The model under review builds one solid part; all positions refer to its coordinate system, in mm. Face numbers are marked on the shaded views. A direction names the side the tool comes from. Give positions to 0.01 mm unless a question says otherwise; leave off trailing zeros. Loops run counter-clockwise (first coordinate to the right, second up) from the corner with the lowest first, then second, coordinate; pieces in that order, holes last. Notation, with made-up numbers: (30.25, -26) - (51.25, -26) arc R20 cw to (51.25, -3) - close; hole circle Ø7 at (55.5, 19). An arc over 180 degrees is marked (long way). Answer as a JSON object with one key per item and string values.
from build123d import *

# Parameters (mm, degrees)
BOSS_EXTRUDE1_DEPTH = 100
SKETCH3_W           = 6
SKETCH3_H           = 6
BOSS_EXTRUDE2_DEPTH = 6
SKETCH4_R           = 1
CUT_EXTRUDE2_DEPTH  = 10
SKETCH5_R           = 1
CUT_EXTRUDE3_DEPTH  = 10
FILLET1_R           = 1
FILLET2_R           = 2
SKETCH7_W           = 11
SKETCH7_H           = 5.6
CUT_EXTRUDE4_DEPTH  = 10
SKETCH13_W          = 6
SKETCH13_H          = 6
BOSS_EXTRUDE3_DEPTH = 6
SKETCH14_R          = 1
CUT_EXTRUDE7_DEPTH  = 6
SKETCH16_R          = 1
CUT_EXTRUDE8_DEPTH  = 6
FILLET3_R           = 2
FILLET4_R           = 1
BOSS_EXTRUDE4_DEPTH = 5
BOSS_EXTRUDE5_DEPTH = 5
SKETCH19_W          = 0.937777778
SKETCH19_H          = 14.2
BOSS_EXTRUDE6_DEPTH = 10
SKETCH20_W          = 0.937777778
SKETCH20_H          = 14.2
BOSS_EXTRUDE7_DEPTH = 10
SKETCH21_W          = 2
SKETCH21_H          = 2.5
BOSS_EXTRUDE8_DEPTH = 1
SKETCH22_W          = 2
SKETCH22_H          = 2.5
BOSS_EXTRUDE9_DEPTH = 1


with BuildPart() as part:
    # Sketch1 → Boss-Extrude1 (new body)
    with BuildSketch(Plane.XY):
        Polygon((0, 0), (10, 0), (2, 45), (0, 45), align=None)
    extrude(amount=BOSS_EXTRUDE1_DEPTH)

    # Sketch3 → Boss-Extrude2 (add)
    with BuildSketch(Plane.ZY):
        with Locations((15.5, 10.1)):
            Rectangle(SKETCH3_W, SKETCH3_H)
        with Locations((84.5, 10.1)):
            Rectangle(SKETCH3_W, SKETCH3_H)
    extrude(amount=BOSS_EXTRUDE2_DEPTH)

    # Sketch4 → Cut-Extrude2 (cut)
    with BuildSketch(Plane(origin=(0, 13.1, 0), x_dir=(1, 0, 0), z_dir=(0, 1, 0))):
        with Locations((-3, -84.5)):
            Circle(SKETCH4_R)
    extrude(amount=-CUT_EXTRUDE2_DEPTH, mode=Mode.SUBTRACT)

    # Sketch5 → Cut-Extrude3 (cut)
    with BuildSketch(Plane(origin=(0, 13.1, 0), x_dir=(1, 0, 0), z_dir=(0, 1, 0))):
        with Locations((-3, -15.5)):
            Circle(SKETCH5_R)
    extrude(amount=-CUT_EXTRUDE3_DEPTH, mode=Mode.SUBTRACT)

    # Fillet1
    fillet1_edges = [part.edges().sort_by_distance(p)[0] for p in [
        (0, 10.1, 12.5),
        (0, 10.1, 18.5),
        (0, 10.1, 87.5),
        (0, 10.1, 81.5),
    ]]
    fillet(fillet1_edges, radius=FILLET1_R)

    # Fillet2
    fillet2_edges = [part.edges().sort_by_distance(p)[0] for p in [
        (-6, 10.1, 12.5),
        (-6, 10.1, 18.5),
        (-6, 10.1, 87.5),
        (-6, 10.1, 81.5),
    ]]
    fillet(fillet2_edges, radius=FILLET2_R)

    # Sketch7 → Cut-Extrude4 (cut)
    with BuildSketch(Plane.ZY):
        with Locations((20.5, 37.8)):
            Rectangle(SKETCH7_W, SKETCH7_H)
        with Locations((79.5, 37.8)):
            Rectangle(SKETCH7_W, SKETCH7_H)
    extrude(amount=-CUT_EXTRUDE4_DEPTH, mode=Mode.SUBTRACT)

    # Sketch13 → Boss-Extrude3 (add)
    with BuildSketch(Plane.ZY):
        with Locations((3, 29.8)):
            Rectangle(SKETCH13_W, SKETCH13_H)
        with Locations((97, 29.8)):
            Rectangle(SKETCH13_W, SKETCH13_H)
    extrude(amount=BOSS_EXTRUDE3_DEPTH)

    # Sketch14 → Cut-Extrude7 (cut)
    with BuildSketch(Plane(origin=(0, 32.8, 0), x_dir=(1, 0, 0), z_dir=(0, 1, 0))):
        with Locations((-3, -3)):
            Circle(SKETCH14_R)
    extrude(amount=-CUT_EXTRUDE7_DEPTH, mode=Mode.SUBTRACT)

    # Sketch16 → Cut-Extrude8 (cut)
    with BuildSketch(Plane(origin=(0, 32.8, 0), x_dir=(1, 0, 0), z_dir=(0, 1, 0))):
        with Locations((-3, -97)):
            Circle(SKETCH16_R)
    extrude(amount=-CUT_EXTRUDE8_DEPTH, mode=Mode.SUBTRACT)

    # Fillet3
    fillet3_edges = [part.edges().sort_by_distance(p)[0] for p in [
        (-6, 29.8, 0),
        (-6, 29.8, 6),
        (-6, 29.8, 94),
        (-6, 29.8, 100),
    ]]
    fillet(fillet3_edges, radius=FILLET3_R)

    # Fillet4
    fillet4_edges = [part.edges().sort_by_distance(p)[0] for p in [
        (0, 29.8, 6),
        (0, 29.8, 94),
    ]]
    fillet(fillet4_edges, radius=FILLET4_R)

    # Sketch17 → Boss-Extrude4 (add)
    with BuildSketch(Plane.ZY):
        Polygon((15, 35), (13.4, 35), (13.4, 42.2), (15, 42.2), (27.6, 42.2), (27.6, 35), (26, 35), (26, 40.6), (15, 40.6), align=None)
        Polygon((74, 35), (72.4, 35), (72.4, 42.2), (74, 42.2), (86.6, 42.2), (86.6, 35), (85, 35), (85, 40.6), (74, 40.6), align=None)
    extrude(amount=-BOSS_EXTRUDE4_DEPTH)

    # Sketch18 → Boss-Extrude5 (add)
    with BuildSketch(Plane.ZY):
        Polygon((15, 35), (13.4, 35), (13.4, 33.4), (27.6, 33.4), (27.6, 35), (26, 35), align=None)
        Polygon((74, 35), (72.4, 35), (72.4, 33.4), (86.6, 33.4), (86.6, 35), (85, 35), align=None)
    extrude(amount=-BOSS_EXTRUDE5_DEPTH)

    # Sketch19 → Boss-Extrude6 (add)
    with BuildSketch(Plane.XZ.offset(-33.4)):
        with Locations((4.531111111, 79.5)):
            Rectangle(SKETCH19_W, SKETCH19_H)
    extrude(amount=BOSS_EXTRUDE6_DEPTH)

    # Sketch20 → Boss-Extrude7 (add)
    with BuildSketch(Plane.XZ.offset(-33.4)):
        with Locations((4.531111111, 20.5)):
            Rectangle(SKETCH20_W, SKETCH20_H)
    extrude(amount=BOSS_EXTRUDE7_DEPTH)

    # Sketch21 → Boss-Extrude8 (add)
    with BuildSketch(Plane.XZ.offset(-40.6)):
        with Locations((4, 83.75)):
            Rectangle(SKETCH21_W, SKETCH21_H)
        with Locations((4, 75.25)):
            Rectangle(SKETCH21_W, SKETCH21_H)
    extrude(amount=BOSS_EXTRUDE8_DEPTH)

    # Sketch22 → Boss-Extrude9 (add)
    with BuildSketch(Plane.XZ.offset(-40.6)):
        with Locations((4, 16.25)):
            Rectangle(SKETCH22_W, SKETCH22_H)
        with Locations((4, 24.75)):
            Rectangle(SKETCH22_W, SKETCH22_H)
    extrude(amount=BOSS_EXTRUDE9_DEPTH)


solid = part.part
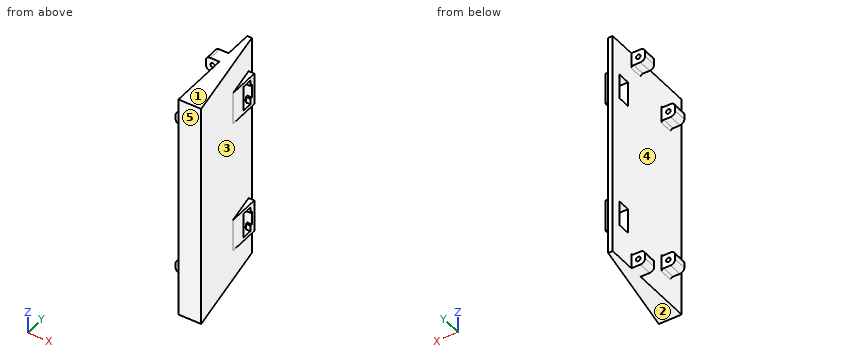
Q1. To check wall thickness, follow probe 1 along Z at (x, y) = (-3, 9.4); probe 2 along Z at (x, y) = (-3, 30.15); probe 3 along Y at (x, z) = (3, 77.5). State the ranges of each line that lie inside material, in increasing order. Write a range as [from, to].
Results:
{"probe 1": "z = [12.5, 14.5], [16.5, 18.5], [81.5, 83.5], [85.5, 87.5]", "probe 2": "z = [0, 2], [4, 6], [94, 96], [98, 100]", "probe 3": "y = [0, 35], [40.6, 42.2]"}
Q2. Clearance check with flat-ended pins moving along their axes: pin 1 Ø1.5 at (x, y) = (-2.5, 9.5) entering from +Z; pin 2 Ø3 at (x, z) = (-3, 97) entering from -Y; pin 3 Ø1.2 at (x, z) = (-3, 15.5) entering from -Y; pin 4 Ø2 at (x, y) = (4.5, 34) entering from +Z. State where each tip first meets the part, or that it passes through.
Results:
{"pin 1": "stops at z = 87.5", "pin 2": "stops at y = 26.8", "pin 3": "passes through", "pin 4": "stops at z = 100"}
Q3. For the marked faces 4 and 5, list the 3-axis set-ups (+Z, -Z, +X, -X, +Y, -Y) from which the entire face can be reached by the end or side of a thin tool; tool diameter is ignored.
Results:
{"face 4": "-X", "face 5": "+Z, -Z, +X, -X, -Y"}
Q4. Consider section C-C, the plane y = 10. State the section outline as (x, z) points.
Results:
{"outline": "(-6, 14.5) arc R2 ccw to (-4, 12.5) - (-1, 12.5) arc R1 cw to (0, 11.5) - (0, 0) - (8.22, 0) - (8.22, 100) - (0, 100) - (0, 88.5) arc R1 cw to (-1, 87.5) - (-4, 87.5) arc R2 ccw to (-6, 85.5) - (-6, 83.5) arc R2 ccw to (-4, 81.5) - (-1, 81.5) arc R1 cw to (0, 80.5) - (0, 19.5) arc R1 cw to (-1, 18.5) - (-4, 18.5) arc R2 ccw to (-6, 16.5) - close; hole circle Ø2 at (-3, 15.5); hole circle Ø2 at (-3, 84.5)"}
Q5. Consider section D-D, the plane z = 51.5. State the section outline as (x, y) points, plus the area to 3 significant figures.
Results:
{"outline": "(0, 0) - (10, 0) - (2, 45) - (0, 45) - close", "area": "270 mm^2"}
Q6. Consider section B-B, the plane x = -3. State how many separate pieces and enclosed holes the cut face has, plus the area to 3 significant figures.
Results:
{"separate pieces": "8", "enclosed holes": "0", "area": "96.0 mm^2"}
Q7. The part is to be moulded in two halves that separate along Z. For the marked faces 1, 2 and 3, say which applies: +Z half, -Z half, draft (parallel to the pull), parting line (faces both ways), or undercut.
Results:
{"face 1": "+Z half", "face 2": "-Z half", "face 3": "undercut"}
Q8. Consider section A-A, the plane z = 3. State the section outline as (x, y) points, plus the area to 3 significant figures.
Results:
{"outline": "(-6, 26.8) - (-4, 26.8) - (-4, 32.8) - (-6, 32.8) - close; (-2, 26.8) - (0, 26.8) - (0, 0) - (10, 0) - (2, 45) - (0, 45) - (0, 32.8) - (-2, 32.8) - close", "area": "294 mm^2"}
